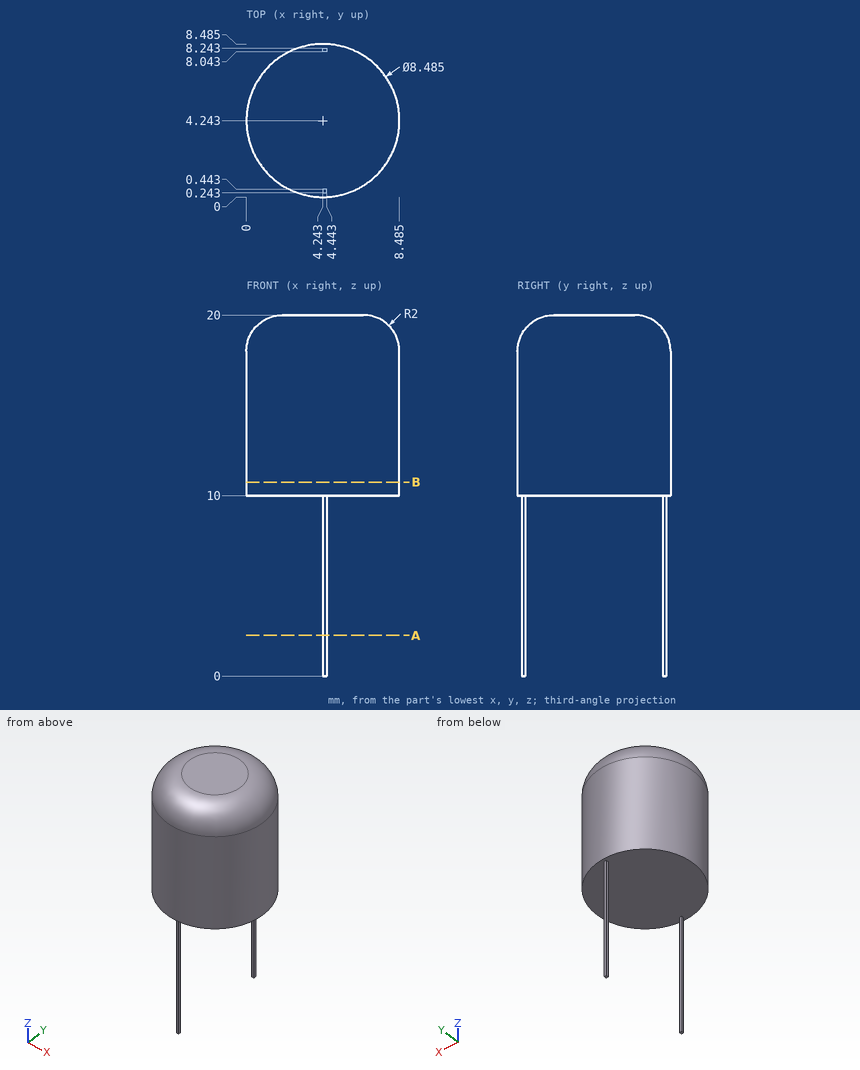
Verification items for this drawing (mm, ordinates from the low corner). Round coordinates to 2 decimals unless told otherwise and drop trailing zeros. Order: outer loops, then holes, each group sorted by start corner. A loop starts at its lowest first (then second) coordinate and runs counter-clockwise, first axis right, second up. Notation, with made-up numbers: (-1.75, -13.5) - (29.25, -13.5) arc R32 ccw to (29.25, 16.5) - close; hole circle Ø4 at (-38, -28.5). An arc over 180 degrees is marked (long way). Use CSV: the item, a comma, the result in double quotes. Start each with the question number.
1) Thickness scan on L1, parallel to Z at x = 1.5, y = 3.75 (1 decimal); L2, parallel to Z at x = 1.5, y = 5.5 (1 decimal); L3, parallel to X at y = 3.5, z = 11.5 (1 decimal). Record the ranges inside material, lowest first.
2) Go/stop test with flat-tipped pins: P1, Ø4, axis at y = 2.5, z = 6, coming from the +X side; P2, Ø1, axis at x = 7, y = 3, coming from the +Z side; P3, Ø1.5, axis at x = 2, z = 18, coming from the +Y side; P4, Ø1, axis at x = 1, z = 14.5, coming from the -Y side (1 decimal). Record where each tip stops, or that it passes through.
3) Section check A-A, the plane z = 2.25. Record the cut outline in (x, y).
4) Section check B-B, the plane z = 10.75. Record the cut outline in (x, y) (1 decimal).
Answers:
1,L1,"z = 10 to 19.9"
1,L2,"z = 10 to 19.8"
1,L3,"x = 0.1 to 8.4"
2,P1,"passes through"
2,P2,"stops at z = 19.98"
2,P3,"stops at y = 8.21"
2,P4,"stops at y = 1"
3,outline,"(4.24, 0.24) - (4.44, 0.24) - (4.44, 0.44) - (4.24, 0.44) - close; (4.24, 8.04) - (4.44, 8.04) - (4.44, 8.24) - (4.24, 8.24) - close"
4,outline,"circle Ø8.5 at (4.2, 4.2)"
